Model file for the job. Use its own axes, mm. A direction names the side the tool comes from. Round coordinates to 2 decimals unless told otherwise and drop trailing zeros. Write each loop counter-clockwise with the first axis right and the second up, starting at its lowest first coordinate (ties: lowest second). Pieces come first, ordered by that corner, then holes. Notation, with made-up numbers: (14, 81) - (59, 81) arc R23 ccw to (59, 101) - close; hole circle Ø1 at (-5.5, 27.5). An arc over 180 degrees is marked (long way). Answer as a JSON object with one key per item and string values. Group by question number.
from build123d import *

# Parameters (mm, degrees)
SKETCH1_R           = 11
BOSS_EXTRUDE1_DEPTH = 50
SKETCH2_W           = 28
SKETCH2_H           = 6
BOSS_EXTRUDE2_DEPTH = 68
SKETCH3_W           = 12
SKETCH3_H           = 50
BOSS_EXTRUDE3_DEPTH = 68
SKETCH4_W           = 28
SKETCH4_H           = 62
BOSS_EXTRUDE4_DEPTH = 12
SKETCH5_W           = 28
SKETCH5_H           = 12
BOSS_EXTRUDE5_DEPTH = 5
CUT_EXTRUDE1_DEPTH  = 122.49490099


with BuildPart() as part:
    # Sketch1 → Boss-Extrude1 (new body)
    with BuildSketch(Plane.XY):
        with BuildLine():
            Line((0, 22), (25.453659816, 22))
            Line((25.453659816, 22), (25.453659816, -40))
            ThreePointArc((25.453659816, -40), (20.193625944, -38.302879135), (16.917350568, -33.851565259))
            ThreePointArc((16.917350568, -33.851565259), (10.327830718, -25.257682927), (0, -22))
            ThreePointArc((0, -22), (-22, 0), (0, 22))
        make_face()
        Circle(SKETCH1_R, mode=Mode.SUBTRACT)
    extrude(amount=-BOSS_EXTRUDE1_DEPTH)

    # Sketch2 → Boss-Extrude2 (add)
    with BuildSketch(Plane(origin=(25.453659816, 0, 0), x_dir=(0, 0, -1), z_dir=(1, 0, 0))):
        with Locations((25, 19)):
            Rectangle(SKETCH2_W, SKETCH2_H)
        with Locations((25, -37)):
            Rectangle(SKETCH2_W, SKETCH2_H)
    extrude(amount=BOSS_EXTRUDE2_DEPTH)

    # Sketch3 → Boss-Extrude3 (add)
    with BuildSketch(Plane(origin=(25.453659816, 0, 0), x_dir=(0, 0, -1), z_dir=(1, 0, 0))):
        with Locations((25, -9)):
            Rectangle(SKETCH3_W, SKETCH3_H)
    extrude(amount=BOSS_EXTRUDE3_DEPTH)

    # Sketch4 → Boss-Extrude4 (add)
    with BuildSketch(Plane(origin=(93.453659816, 0, 0), x_dir=(0, 0, -1), z_dir=(1, 0, 0))):
        with Locations((25, -9)):
            Rectangle(SKETCH4_W, SKETCH4_H)
    extrude(amount=BOSS_EXTRUDE4_DEPTH)

    # Sketch5 → Boss-Extrude5 (add)
    with BuildSketch(Plane(origin=(105.453659816, 0, 0), x_dir=(0, 0, -1), z_dir=(1, 0, 0))):
        with Locations((25, 16)):
            Rectangle(SKETCH5_W, SKETCH5_H)
        with Locations((25, -34)):
            Rectangle(SKETCH5_W, SKETCH5_H)
    extrude(amount=BOSS_EXTRUDE5_DEPTH)

    # Sketch8 → Cut-Extrude1 (cut, through all)
    with BuildSketch(Plane.XY.offset(-19)):
        with BuildLine():
            Line((50.453659816, -1), (68.453659816, -1))
            ThreePointArc((68.453659816, -1), (76.453659816, -9), (68.453659816, -17))
            Line((68.453659816, -17), (50.453659816, -17))
            ThreePointArc((50.453659816, -17), (42.453659816, -9), (50.453659816, -1))
        make_face()
    extrude(amount=-CUT_EXTRUDE1_DEPTH, mode=Mode.SUBTRACT)


solid = part.part
(1) Slice it at C-C (y = -9). Write the cut outline in (x, z), then the cut area to 3 significant figures.
(2) 3-axis set-ups, long thin cutter, end or side, ignore diameter. For faces 4 (the flat face through (60, -17, -25)), 5 (the flat face through (93.454, -9, -15)), 6 (the flat face through (105.454, -9, -25)): which of +Z, -Z, +X, -X, +Y, -Y reach the whole face in a straight line?
(3) Pull direction Y, two halves, no side cores. Call faces 1 (the flat face through (96, -9, -11)), 2 (the flat face through (59, -1, -25)), 3 (the cylindrical face through (-22, 0, -25)): pulls with the +Y half, pulls with the -Y half, needs draft (parallel to the pull), parting line crosses it, or undercut.
(4) Slice it at B-B (z = -34.5). Write the cut outline in (x, y).
(5) Slice it at A-A (x = 72). Write the cut outline in (y, z).
(6) Slice it at D-D (z = -5). Write the cut outline in (x, y).
(7) Flat gauge pins, fed straight in: pin 1 (3 mm diameter, centred on x = 62.5, y = 5, fed in from +Z); pin 2 (5 mm diameter, centred on y = -19, z = -19, fed in from -X); pin 3 (1.5 mm diameter, centred on y = -16, z = -14, fed in from +X). Where does each tip first touch, or does it go through?
(8) Drill centre lines: line 1 (Y direction, x = 89.5, z = -11.5); line 2 (X direction, y = -9, z = -25.5); line 3 (Z direction, x = 62, y = 13). Where is each one in solid material? Low to high. Write a range as from..to.
Answer:
{
 "1": {"outline": "(-20.07, -50) - (-6.32, -50) - (-6.32, 0) - (-20.07, 0) - close; (6.32, -50) - (25.45, -50) - (25.45, -31) - (42.45, -31) - (42.45, -19) - (25.45, -19) - (25.45, 0) - (6.32, 0) - close; (76.45, -31) - (93.45, -31) - (93.45, -39) - (105.45, -39) - (105.45, -11) - (93.45, -11) - (93.45, -19) - (76.45, -19) - close", "area": "2,390 mm²"},
 "2": {"face 4": "+Z, -Z", "face 5": "+Z", "face 6": "+Z, -Z, +X"},
 "3": {"face 1": "needs draft", "face 2": "undercut", "face 3": "parting line crosses it"},
 "4": {"outline": "(0, -22) arc R18 cw to (16.92, -33.85) arc R9 ccw to (25.45, -40) - (110.45, -40) - (110.45, -28) - (105.45, -28) - (105.45, 10) - (110.45, 10) - (110.45, 22) - (0, 22) arc R22 ccw to start; hole circle Ø22 at (0, 0); hole (25.45, -34) - (93.45, -34) - (93.45, 16) - (25.45, 16) - close"},
 "5": {"outline": "(-40, -39) - (-34, -39) - (-34, -31) - (-16.17, -31) - (-16.17, -19) - (-34, -19) - (-34, -11) - (-40, -11) - close; (-1.83, -31) - (16, -31) - (16, -39) - (22, -39) - (22, -11) - (16, -11) - (16, -19) - (-1.83, -19) - close"},
 "6": {"outline": "(0, -22) arc R18 cw to (16.92, -33.85) arc R9 ccw to (25.45, -40) - (25.45, 22) - (0, 22) arc R22 ccw to start; hole circle Ø22 at (0, 0)"},
 "7": {"pin 1": "z = -19", "pin 2": "x = -14.55", "pin 3": "x = 105.45"},
 "8": {"line 1": "-40..-34, 16..22", "line 2": "-20.07..-6.32, 6.32..42.45, 76.45..105.45", "line 3": "-31..-19"}
}
